Could you check a few things on this drawing? It's one solid part, dimensions in mm from its lowest x, y, z. A direction names the side the tool comes from. Give positions to 0.01 mm unless a question says otherwise; leave off trailing zeros. Order: outer loops, then holes, each group sorted by start corner. A loop starts at its lowest first (then second) coordinate and runs counter-clockwise, first axis right, second up.
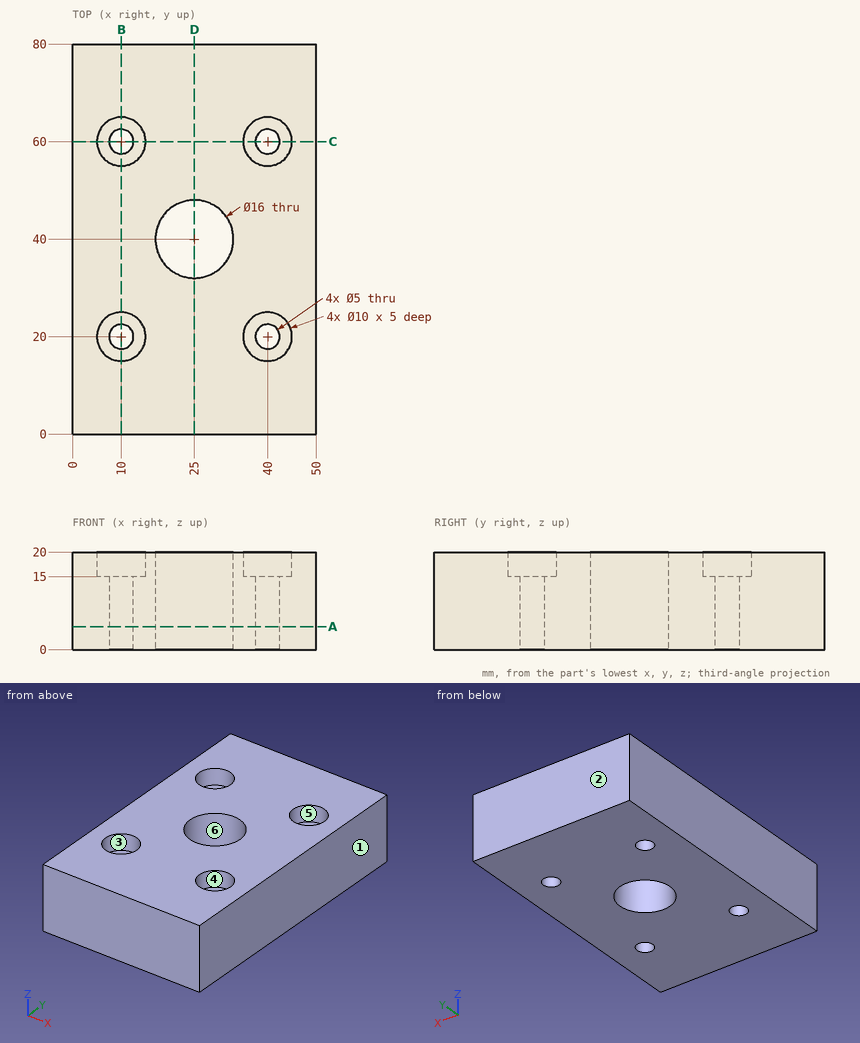
Q1. I need wall thicknesses on L1, parallel to Y at x = 10, z = 17.2; L2, parallel to Y at x = 40, z = 9; L3, parallel to X at y = 62, z = 9. Which ranges of each line are inside material? Lowest first, please.
Filled sheet:
L1: y = 0 to 15, 25 to 55, 65 to 80
L2: y = 0 to 17.5, 22.5 to 57.5, 62.5 to 80
L3: x = 0 to 8.5, 11.5 to 38.5, 41.5 to 50
Q2. If we section it at A-A on z = 4.75: List the corners of the cut face in (x, y) for me.
Filled sheet:
outline: (0, 0) - (50, 0) - (50, 80) - (0, 80) - close; hole circle Ø5 at (10, 20); hole circle Ø5 at (10, 60); hole circle Ø16 at (25, 40); hole circle Ø5 at (40, 20); hole circle Ø5 at (40, 60)
Q3. For the marked faces 5 and 6, which set-ups out of +Z, -Z, +X, -X, +Y, -Y let a thin tool reach every point of the face, with its end or its side?
Filled sheet:
face 5: +Z
face 6: +Z, -Z
Q4. If we section it at D-D on x = 25: List the corners of the cut face in (y, z) for me.
Filled sheet:
outline: (0, 0) - (32, 0) - (32, 20) - (0, 20) - close; (48, 0) - (80, 0) - (80, 20) - (48, 20) - close
Q5. If we section it at B-B on x = 10: List the corners of the cut face in (y, z) for me.
Filled sheet:
outline: (0, 0) - (17.5, 0) - (17.5, 15) - (15, 15) - (15, 20) - (0, 20) - close; (22.5, 0) - (57.5, 0) - (57.5, 15) - (55, 15) - (55, 20) - (25, 20) - (25, 15) - (22.5, 15) - close; (62.5, 0) - (80, 0) - (80, 20) - (65, 20) - (65, 15) - (62.5, 15) - close
Q6. Thinking about a two-plate mould opening in Y: for the marked faces 1, 2, 3 and 4, which applies, released by +Y, released by -Y, zero draft, split by the parting line, or undercut?
Filled sheet:
face 1: zero draft
face 2: released by +Y
face 3: undercut
face 4: undercut
Q7. I'm going to push flat-ended pins straight in: P1, Ø6, axis at x = 10, y = 60, coming from the +Z side; P2, Ø3, axis at x = 40, y = 60, coming from the +Z side. Where does each tip first touch, or does it pass through?
Filled sheet:
P1: stops at z = 15
P2: passes through
Q8. If we section it at C-C on y = 60: List the corners of the cut face in (x, z) for me.
Filled sheet:
outline: (0, 0) - (7.5, 0) - (7.5, 15) - (5, 15) - (5, 20) - (0, 20) - close; (12.5, 0) - (37.5, 0) - (37.5, 15) - (35, 15) - (35, 20) - (15, 20) - (15, 15) - (12.5, 15) - close; (42.5, 0) - (50, 0) - (50, 20) - (45, 20) - (45, 15) - (42.5, 15) - close
